Read the model definition and answer for the solid it produces. Units are mm, in the model's axes. A direction names the side the tool comes from. Round coordinates to 2 decimals unless told otherwise and drop trailing zeros. Write each loop counter-clockwise with the first axis right and the second up, starting at its lowest first coordinate (ties: lowest second). Pieces come first, ordered by that corner, then holes.
from build123d import *

# Parameters (mm, degrees)
SKETCH1_W               = 40
SKETCH1_H               = 105
BOSS_EXTRUDE3_DEPTH     = 75
SKETCH4_W               = 97
SKETCH4_H               = 71
CUT_EXTRUDE2_DEPTH      = 36
SKETCH5_W               = 40
SKETCH5_H               = 9.8
CUT_EXTRUDE3_DEPTH      = 2
SKETCH6_W               = 40
SKETCH6_H               = 9.8
CUT_EXTRUDE4_DEPTH      = 2
SKETCH7_W               = 101
SKETCH7_H               = 9.8
CUT_EXTRUDE5_DEPTH      = 2
SKETCH8_R               = 1.55
CUT_EXTRUDE6_DEPTH      = 102
CUT_EXTRUDE6_DEPTH_BACK = 5
SKETCH9_W               = 8
SKETCH9_H               = 10
CUT_EXTRUDE7_DEPTH      = 2
SKETCH10_R              = 1.55
CUT_EXTRUDE8_DEPTH      = 2
SKETCH11_W              = 8
SKETCH11_H              = 10
CUT_EXTRUDE9_DEPTH      = 2
CUT_EXTRUDE10_REACH     = 42
SKETCH12_W              = 20
SKETCH12_H              = 40


with BuildPart() as part:
    # Sketch1 → Boss-Extrude3 (new body)
    with BuildSketch(Plane(origin=(0, 0, 0), x_dir=(1, 0, 0), z_dir=(0, 1, 0))):
        Rectangle(SKETCH1_W, SKETCH1_H)
    extrude(amount=BOSS_EXTRUDE3_DEPTH)

    # Sketch4 → Cut-Extrude2 (cut)
    with BuildSketch(Plane(origin=(20, 0, 0), x_dir=(0, 0, -1), z_dir=(1, 0, 0))):
        with Locations((0, 39.5)):
            Rectangle(SKETCH4_W, SKETCH4_H)
    extrude(amount=-CUT_EXTRUDE2_DEPTH, mode=Mode.SUBTRACT)

    # Sketch5 → Cut-Extrude3 (cut)
    with BuildSketch(Plane.XY.offset(52.5)):
        with Locations((0, 70.1)):
            Rectangle(SKETCH5_W, SKETCH5_H)
    extrude(amount=-CUT_EXTRUDE3_DEPTH, mode=Mode.SUBTRACT)

    # Sketch6 → Cut-Extrude4 (cut)
    with BuildSketch(Plane(origin=(0, 0, -52.5), x_dir=(-1, 0, 0), z_dir=(0, 0, -1))):
        with Locations((0, 70.1)):
            Rectangle(SKETCH6_W, SKETCH6_H)
    extrude(amount=-CUT_EXTRUDE4_DEPTH, mode=Mode.SUBTRACT)

    # Sketch7 → Cut-Extrude5 (cut)
    with BuildSketch(Plane.ZY.offset(20)):
        with Locations((0, 70.1)):
            Rectangle(SKETCH7_W, SKETCH7_H)
    extrude(amount=-CUT_EXTRUDE5_DEPTH, mode=Mode.SUBTRACT)

    # Sketch8 → Cut-Extrude6 (cut, two sides)
    with BuildSketch(Plane(origin=(0, 0, 48.5), x_dir=(-1, 0, 0), z_dir=(0, 0, -1))) as cut_extrude6_sk:
        with Locations((-16, 18)):
            Circle(SKETCH8_R)
        with Locations((-16, 46)):
            Circle(SKETCH8_R)
    extrude(amount=CUT_EXTRUDE6_DEPTH, mode=Mode.SUBTRACT)
    extrude(cut_extrude6_sk.sketch, amount=-CUT_EXTRUDE6_DEPTH_BACK, mode=Mode.SUBTRACT)

    # Sketch9 → Cut-Extrude7 (cut)
    with BuildSketch(Plane(origin=(0, 0, 48.5), x_dir=(-1, 0, 0), z_dir=(0, 0, -1))):
        with Locations((-16, 18)):
            Rectangle(SKETCH9_W, SKETCH9_H)
        with Locations((-16, 46)):
            Rectangle(SKETCH9_W, SKETCH9_H)
    extrude(amount=-CUT_EXTRUDE7_DEPTH, mode=Mode.SUBTRACT)

    # Sketch10 → Cut-Extrude8 (cut)
    with BuildSketch(Plane.ZY.offset(18)):
        with Locations((0, 71)):
            Circle(SKETCH10_R)
    extrude(amount=-CUT_EXTRUDE8_DEPTH, mode=Mode.SUBTRACT)

    # Sketch11 → Cut-Extrude9 (cut)
    with BuildSketch(Plane.XY.offset(-48.5)):
        with Locations((16, 46)):
            Rectangle(SKETCH11_W, SKETCH11_H)
        with Locations((16, 18)):
            Rectangle(SKETCH11_W, SKETCH11_H)
    extrude(amount=-CUT_EXTRUDE9_DEPTH, mode=Mode.SUBTRACT)

    # Sketch12 → Cut-Extrude10 (cut, up to next)
    with BuildSketch(Plane.ZY.offset(20), mode=Mode.PRIVATE) as cut_extrude10_sk1:
        with Locations((-33, 44)):
            Rectangle(SKETCH12_W, SKETCH12_H)
    cut_extrude10_tool1 = extrude(cut_extrude10_sk1.sketch, amount=-CUT_EXTRUDE10_REACH, mode=Mode.PRIVATE) & part.part
    add(cut_extrude10_tool1.solids().sort_by_distance((-20, 44, -33))[0], mode=Mode.SUBTRACT)
    # Sketch12 → Cut-Extrude10 (cut, up to next)
    with BuildSketch(Plane.ZY.offset(20), mode=Mode.PRIVATE) as cut_extrude10_sk2:
        with Locations((-11, 44)):
            Rectangle(SKETCH12_W, SKETCH12_H)
    cut_extrude10_tool2 = extrude(cut_extrude10_sk2.sketch, amount=-CUT_EXTRUDE10_REACH, mode=Mode.PRIVATE) & part.part
    add(cut_extrude10_tool2.solids().sort_by_distance((-20, 44, -11))[0], mode=Mode.SUBTRACT)
    # Sketch12 → Cut-Extrude10 (cut, up to next)
    with BuildSketch(Plane.ZY.offset(20), mode=Mode.PRIVATE) as cut_extrude10_sk3:
        with Locations((11, 44)):
            Rectangle(SKETCH12_W, SKETCH12_H)
    cut_extrude10_tool3 = extrude(cut_extrude10_sk3.sketch, amount=-CUT_EXTRUDE10_REACH, mode=Mode.PRIVATE) & part.part
    add(cut_extrude10_tool3.solids().sort_by_distance((-20, 44, 11))[0], mode=Mode.SUBTRACT)
    # Sketch12 → Cut-Extrude10 (cut, up to next)
    with BuildSketch(Plane.ZY.offset(20), mode=Mode.PRIVATE) as cut_extrude10_sk4:
        with Locations((33, 44)):
            Rectangle(SKETCH12_W, SKETCH12_H)
    cut_extrude10_tool4 = extrude(cut_extrude10_sk4.sketch, amount=-CUT_EXTRUDE10_REACH, mode=Mode.PRIVATE) & part.part
    add(cut_extrude10_tool4.solids().sort_by_distance((-20, 44, 33))[0], mode=Mode.SUBTRACT)


solid = part.part
Q1. Determine the mould class of faces 1 (the flat face through (18, 18, -50.5)), 2 (the flat face through (-18, 69, -1)), 3 (the cylindrical face through (16.202, 19.537, 51.486)) for opening direction X: pulls with the +X half, pulls with the -X half, needs draft (parallel to the pull), parting line crosses it, or undercut.
Verdict:
face 1: needs draft
face 2: pulls with the -X half
face 3: undercut
Q2. Section A-A (y = 71) is taken. Determine the outline of the cut face in (x, z), then the cut area to 3 significant figures.
Verdict:
outline: (-18, -50.5) - (20, -50.5) - (20, -48.5) - (-16, -48.5) - (-16, -1.55) - (-18, -1.55) - close; (-18, 1.55) - (-16, 1.55) - (-16, 48.5) - (20, 48.5) - (20, 50.5) - (-18, 50.5) - close
area: 340 mm2
Q3. Which of the six approach directions +Z, -Z, +X, -X, +Y, -Y give full straight-line access (tool end or side, diameter ignored) to faces 4 (the flat face through (-18, 24, -33)), 5 (the flat face through (1, 70, 50.5)), 6 (the flat face through (18, 46, -50.5)), 7 (the flat face through (2, 39, 48.5)), 8 (the flat face through (0, 32, 52.5))?
Verdict:
face 4: +X, -X
face 5: +Z, +X, -X, +Y
face 6: +X
face 7: +X, +Y
face 8: +Z, +X, -X, +Y, -Y
Q4. Section B-B (z = 36) is taken. Determine the outline of the cut face in (x, y), then the cut area to 3 significant figures.
Verdict:
outline: (-20, 0) - (20, 0) - (20, 4) - (-16, 4) - (-16, 24) - (-20, 24) - close; (-20, 64) - (-16, 64) - (-16, 75) - (-18, 75) - (-18, 65.2) - (-20, 65.2) - close
area: 264 mm2
Q5. Section D-D (x = 6.5) is taken. Determine the outline of the cut face in (y, z).
Verdict:
outline: (0, -52.5) - (65.2, -52.5) - (65.2, -50.5) - (75, -50.5) - (75, -48.5) - (4, -48.5) - (4, 48.5) - (75, 48.5) - (75, 50.5) - (65.2, 50.5) - (65.2, 52.5) - (0, 52.5) - close
Q6. Section C-C (y = 27) is taken. Determine the outline of the cut face in (x, z), then the cut area to 3 significant figures.
Verdict:
outline: (-20, -52.5) - (20, -52.5) - (20, -48.5) - (-16, -48.5) - (-16, -43) - (-20, -43) - close; (-20, -23) - (-16, -23) - (-16, -21) - (-20, -21) - close; (-20, -1) - (-16, -1) - (-16, 1) - (-20, 1) - close; (-20, 21) - (-16, 21) - (-16, 23) - (-20, 23) - close; (-20, 43) - (-16, 43) - (-16, 48.5) - (20, 48.5) - (20, 52.5) - (-20, 52.5) - close
area: 388 mm2
Q7. Flat-ended cylindrical pins translate along their axes: pin 1 Ø1 at (x, z) = (-6, 3.5) entering from +Y; pin 2 Ø3 at (x, y) = (16, 18) entering from +Z; pin 3 Ø1 at (y, z) = (48, -49.5) entering from +X. Find the tip coordinate at first contact, or state that the pin passes through.
Verdict:
pin 1: stops at y = 4
pin 2: passes through
pin 3: stops at x = 12
Q8. Straight lines are drawn through the part: probe 1 along Y at (x, z) = (16, 51.3); probe 2 along Z at (x, y) = (-18, 61.5); probe 3 along Z at (x, y) = (0, 39). For each, find the intervals that lie inside material, in ascending order.
Verdict:
probe 1: y = 0 to 16.45, 19.55 to 44.45, 47.55 to 65.2
probe 2: z = -52.5 to -43, -23 to -21, -1 to 1, 21 to 23, 43 to 52.5
probe 3: z = -52.5 to -48.5, 48.5 to 52.5
